Model file for the job. Use its own axes, mm. A direction names the side the tool comes from. Give positions to 0.01 mm unless a question says otherwise; leave off trailing zeros. Order: outer loops, then holes, each group sorted by start corner. A loop starts at its lowest first (then second) coordinate and runs counter-clockwise, first axis right, second up. Notation, with made-up numbers: M 1.5,37.25 L 40.5,37.25 A10 cw 40.5,51.25 Z; hole C 0.5,4.5 d4. An arc over 180 degrees is marked long. Return JSON: item names as keys, results as strings. Group by question number.
1. Pin check, flat tips, straight feed: pin 1 (1.5 mm diameter, centred on x = 3, z = 3.5, fed in from +Y); pin 2 (10 mm diameter, centred on x = 25.5, y = -8.5, fed in from -Z); pin 3 (12 mm diameter, centred on y = -24, z = 8.5, fed in from -X). Stop position of each tip, or through.
2. Slice it at C-C on z = 11. List the corners of the cut face in (x, y), then the cut area to 3 significant figures.
3. Slice it at A-A on x = 0. List the corners of the cut face in (y, z).
4. Wall check: probe 1 along Y at (x, z) = (0, 9.5); probe 2 along Z at (x, y) = (-10.5, -3); probe 3 along X at (y, z) = (-2, 5.75). Give the ranges that are in metal, low to high. Write a range as [from, to].
5. 3-axis set-ups, long thin cutter, end or side, ignore diameter. For faces 1 (the face through (-12.6, 37.3, 0)), 2 (the face through (-8.49, -38.23, 11.27)): which of +Z, -Z, +X, -X, +Y, -Y reach the whole face in a straight line?
6. Two-plate mould, pull along X, no slides. Class faces 3 (the face through (-1, 1, 25.4)), 4 (the face through (-1, 1, 22.86)), 5 (the face through (-9.04, -40.71, 10.02)): released by +X, released by -X, zero draft, split by the parting line, or undercut.
from build123d import *

# Parameters (mm, degrees)
F0_R     = 41.701709
F1_DEPTH = 25.4
F2_T     = -2.54
F3_R     = 5.08


with BuildPart() as f1:
    # F0 (on Top) → F1 (new body)
    with BuildSketch(Plane.XY):
        Circle(F0_R)
    extrude(amount=F1_DEPTH)

    # F2
    f2_openings = [f1.faces().sort_by_distance(p)[0] for p in [
        (0, 0, 0),
    ]]
    offset(amount=F2_T, openings=f2_openings)

    # F3
    f3_edges = [f1.edges().sort_by_distance(p)[0] for p in [
        (-41.701709, 0, 25.4),
    ]]
    fillet(f3_edges, radius=F3_R)


solid = f1.part
Result:
{
 "1": {"pin 1": "stops at y = 41.64", "pin 2": "stops at z = 22.86", "pin 3": "stops at x = -37.62"},
 "2": {"outline": "C 0,0 d83.4; hole C 0,0 d78.32", "area": "645 mm2"},
 "3": {"outline": "M -41.7,0 L -39.16,0 L -39.16,22.86 L 39.16,22.86 L 39.16,0 L 41.7,0 L 41.7,20.32 A5.08 ccw 36.62,25.4 L -36.62,25.4 A5.08 ccw -41.7,20.32 Z"},
 "4": {"probe 1": "y = [-41.7, -39.16], [39.16, 41.7]", "probe 2": "z = [22.86, 25.4]", "probe 3": "x = [-41.65, -39.11], [39.11, 41.65]"},
 "5": {"face 1": "-Z, +X, -X, +Y, -Y", "face 2": "-Z"},
 "6": {"face 3": "zero draft", "face 4": "undercut", "face 5": "split by the parting line"}
}
